from build123d import *

# Parameters (mm, degrees)
BOSS_EXTRUDE1_DEPTH      = 2.54
BOSS_EXTRUDE1_DEPTH_BACK = 8.89
SKETCH1_W                = 191.555456122
SKETCH1_H                = 84.203656122
SKETCH1_W_2              = 182.5752
SKETCH1_H_2              = 75.2234
SKETCH3_W                = 182.5752
SKETCH3_H                = 75.2234
BOSS_EXTRUDE4_DEPTH      = 2.54
SKETCH4_R                = 2.9150268
SKETCH4_R_2              = 1.75
BOSS_EXTRUDE6_DEPTH      = 5.842


with BuildPart() as part:
    # Sketch1 → Boss-Extrude1 (new, two sides: drawn at the far end of the back side and taken through both)
    with BuildSketch(Plane.XY.offset(-BOSS_EXTRUDE1_DEPTH_BACK)):
        with Locations((87.6132, 33.6117)):
            Rectangle(SKETCH1_W, SKETCH1_H)
        with Locations((87.6132, 33.6117)):
            Rectangle(SKETCH1_W_2, SKETCH1_H_2, mode=Mode.SUBTRACT)
    extrude(amount=BOSS_EXTRUDE1_DEPTH + BOSS_EXTRUDE1_DEPTH_BACK)

    # Sketch3 → Boss-Extrude4 (add)
    with BuildSketch(Plane(origin=(0, 0, -8.89), x_dir=(-1, 0, 0), z_dir=(0, 0, -1))):
        with Locations((-87.6132, 33.6117)):
            Rectangle(SKETCH3_W, SKETCH3_H)
    extrude(amount=-BOSS_EXTRUDE4_DEPTH)

    # Sketch4 → Boss-Extrude6 (add)
    # profile 1 of 4: a face of its own
    with BuildSketch(Plane.XY.offset(-6.35)):
        with Locations(Location((0.0086, 66.9562, 0), (0, 0, 180))):
            Circle(SKETCH4_R)
        with Locations((0.0086, 66.9562)):
            Circle(SKETCH4_R_2, mode=Mode.SUBTRACT)
    # profile 2 of 4: a face of its own
    with BuildSketch(Plane.XY.offset(-6.35)):
        with Locations(Location((174.7606, 66.9562, 0), (0, 0, 180))):
            Circle(SKETCH4_R)
        with Locations((174.7606, 66.9562)):
            Circle(SKETCH4_R_2, mode=Mode.SUBTRACT)
    # profile 3 of 4: a face of its own
    with BuildSketch(Plane.XY.offset(-6.35)):
        with Locations(Location((174.6, 0, 0), (0, 0, 180))):
            Circle(SKETCH4_R)
        with Locations((174.6, 0)):
            Circle(SKETCH4_R_2, mode=Mode.SUBTRACT)
    # profile 4 of 4: a face of its own
    with BuildSketch(Plane.XY.offset(-6.35)):
        with Locations(Location((0, 0, 0), (0, 0, 180))):
            Circle(SKETCH4_R)
        Circle(SKETCH4_R_2, mode=Mode.SUBTRACT)
    extrude(amount=BOSS_EXTRUDE6_DEPTH)


solid = part.part
CAD build for the part. Positions are in the model's coordinates, mm. A direction names the side the tool comes from. Round coordinates to 2 decimals unless told otherwise and drop trailing zeros. Write each loop counter-clockwise with the first axis right and the second up, starting at its lowest first coordinate (ties: lowest second). Pieces come first, ordered by that corner, then holes. Notation, with made-up numbers: M 71.25,5.5 L 82.25,5.5 A13 cw 82.25,23.5 Z; hole C -17.75,24.25 d6. An arc over 180 degrees is marked long. Use a Markdown table: item, result. Add a question column.
1. Slice it at B-B on z = -3.25. Give the number of separate pieces and of enclosed holes in the cut face, then the cut area to 3 significant figures.
2. Flat gauge pins, fed straight in: P1, Ø1.8, axis at x = 0.5, y = 66.5, coming from the +Z side; P2, Ø4.5, axis at x = -0.5, y = 66, coming from the +Z side. Where does each tip first touch, or does it go through?
3. Slice it at C-C on x = 54. Give the cut face in (y, z).
4. Pull direction X, two halves, no side cores. Call faces 1 (the face through (178.901, 33, -2)), 2 (the face through (1.617, -0.67, -3.47)), 3 (the face through (101, 74, 2.54)), 4 (the face through (-8.165, 33, -3)): released by +X, released by -X, zero draft, split by the parting line, or undercut.
5. 3-axis set-ups, long thin cutter, end or side, ignore diameter. For faces 5 (the face through (2.15, -1.97, -3.47)), 6 (the face through (86, 75.714, -3)): which of +Z, -Z, +X, -X, +Y, -Y reach the whole face in a straight line?
6. Slice it at D-D on y = 9. Give the cut face in (x, z), then the cut area to 3 significant figures.
7. Drill centre lines: probe 1 along Y at (x, z) = (174.6, -4.2); probe 2 along Y at (x, z) = (163.5, -0.75); probe 3 along X at (y, z) = (39, -3.25). Where is each one in solid material? Low to high.
8. Slice it at A-A on y = 0. Give the cut face in (x, z).
Reply:
| question | item | result |
|---|---|---|
| 1 | separate pieces | 5 |
| 1 | enclosed holes | 5 |
| 1 | area | 2,460 mm^2 |
| 2 | P1 | stops at z = -6.35 |
| 2 | P2 | stops at z = -0.51 |
| 3 | outline | M -8.49,-8.89 L 75.71,-8.89 L 75.71,2.54 L 71.22,2.54 L 71.22,-6.35 L -4,-6.35 L -4,2.54 L -8.49,2.54 Z |
| 4 | face 1 | undercut |
| 4 | face 2 | undercut |
| 4 | face 3 | zero draft |
| 4 | face 4 | released by -X |
| 5 | face 5 | +Z |
| 5 | face 6 | +Z, -Z, +X, -X, +Y |
| 6 | outline | M -8.16,-8.89 L 183.39,-8.89 L 183.39,2.54 L 178.9,2.54 L 178.9,-6.35 L -3.67,-6.35 L -3.67,2.54 L -8.16,2.54 Z |
| 6 | area | 566 mm^2 |
| 7 | probe 1 | y = -8.49 to -4, -2.92 to -1.75, 1.75 to 2.92, 64.05 to 65.21, 68.7 to 69.87, 71.22 to 75.71 |
| 7 | probe 2 | y = -8.49 to -4, 71.22 to 75.71 |
| 7 | probe 3 | x = -8.16 to -3.67, 178.9 to 183.39 |
| 8 | outline | M -8.16,-8.89 L 183.39,-8.89 L 183.39,2.54 L 178.9,2.54 L 178.9,-6.35 L 177.52,-6.35 L 177.52,-0.51 L 176.35,-0.51 L 176.35,-6.35 L 172.85,-6.35 L 172.85,-0.51 L 171.68,-0.51 L 171.68,-6.35 L 2.92,-6.35 L 2.92,-0.51 L 1.75,-0.51 L 1.75,-6.35 L -1.75,-6.35 L -1.75,-0.51 L -2.92,-0.51 L -2.92,-6.35 L -3.67,-6.35 L -3.67,2.54 L -8.16,2.54 Z |
